Can you work these out from the drawing? Everything is in mm from the part's minimum corner. Give positions to 0.01 mm unless a question says otherwise; leave off trailing zeros. Write each loop counter-clockwise with the first axis right and the second up, starting at its lowest first coordinate (ties: lowest second). Pieces come first, ordered by that corner, then holes. Notation, with made-up numbers: (61, 55.5) -> (117, 55.5) arc R34 ccw to (117, 86.5) -> close; hole circle Ø4 at (1, 37). An arc over 180 degrees is marked (long way). Use one line per item in the form item = value.
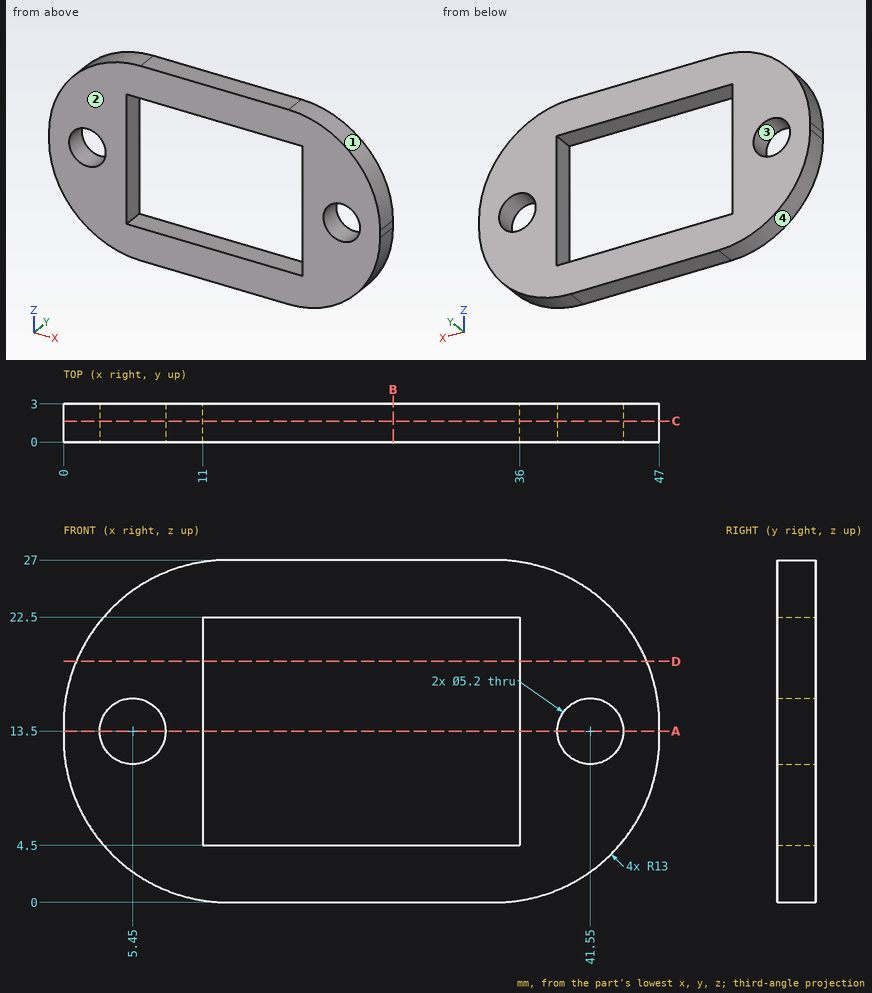
Q1. I want a section at C-C, the plane y = 1.65. Write out the boundary of the cut face in (x, z), and give its area (3 significant figures).
Result set:
outline = (0, 13) arc R13 ccw to (13, 0) -> (34, 0) arc R13 ccw to (47, 13) -> (47, 14) arc R13 ccw to (34, 27) -> (13, 27) arc R13 ccw to (0, 14) -> close; hole circle Ø5.2 at (5.45, 13.5); hole (11, 4.5) -> (36, 4.5) -> (36, 22.5) -> (11, 22.5) -> close; hole circle Ø5.2 at (41.55, 13.5)
area = 631 mm2
Q2. If I drill on line 1 along X through (y, z) = (1.4, 13.5); line 2 along X through (y, z) = (0.8, 12.5); line 3 along Z through (x, y) = (16.5, 0.3), over which ranges is the centre line in solid material (lowest first)? Write a range as from..to.
Result set:
line_1 = 0..2.85, 8.05..11, 36..38.95, 44.15..47
line_2 = 0.01..3.05, 7.85..11, 36..39.15, 43.95..46.99
line_3 = 0..4.5, 22.5..27
Q3. I want a section at B-B, the plane x = 26. Write out the boundary of the cut face in (y, z).
Result set:
outline = (0, 0) -> (3, 0) -> (3, 4.5) -> (0, 4.5) -> close; (0, 22.5) -> (3, 22.5) -> (3, 27) -> (0, 27) -> close
Q4. I want a section at D-D, the plane z = 19. Write out the boundary of the cut face in (x, y), and give its area (3 significant figures).
Result set:
outline = (1, 0) -> (11, 0) -> (11, 3) -> (1, 3) -> close; (36, 0) -> (46, 0) -> (46, 3) -> (36, 3) -> close
area = 60.0 mm2
Q5. Will these pins go through, and if not, where does the flat tip stop? pin 1 Ø4.5 at (x, z) = (41.55, 13.5) entering from +Y; pin 2 Ø0.9 at (y, z) = (1.5, 10.5) entering from +X.
Result set:
pin_1 = through
pin_2 = 46.84
Q6. If we mould it in two halves opening along Z, with no side actions, what happens to the marked faces 1, 2, 3 and 4? For each: +Z half, -Z half, draft (parallel to the pull), parting line (faces both ways), or undercut.
Result set:
face_1 = +Z half
face_2 = draft
face_3 = undercut
face_4 = -Z half
Q7. I want a section at A-A, the plane z = 13.5. Write out the boundary of the cut face in (x, y), and give its area (3 significant figures).
Result set:
outline = (0, 0) -> (2.85, 0) -> (2.85, 3) -> (0, 3) -> close; (8.05, 0) -> (11, 0) -> (11, 3) -> (8.05, 3) -> close; (36, 0) -> (38.95, 0) -> (38.95, 3) -> (36, 3) -> close; (44.15, 0) -> (47, 0) -> (47, 3) -> (44.15, 3) -> close
area = 34.8 mm2
